```python
from build123d import *

# Parameters (mm, degrees)
SKETCH1_W           = 34
SKETCH1_H           = 30
SKETCH1_R           = 2
BOSS_EXTRUDE1_DEPTH = 22
SKETCH3_R           = 4
CUT_EXTRUDE1_DEPTH  = 30


with BuildPart() as part:
    # Sketch1 → Boss-Extrude1 (new body)
    with BuildSketch(Plane.XY):
        Rectangle(SKETCH1_W, SKETCH1_H)
        with Locations((-12, 9)):
            Circle(SKETCH1_R, mode=Mode.SUBTRACT)
        with Locations((-12, -9)):
            Circle(SKETCH1_R, mode=Mode.SUBTRACT)
        with Locations((12, 9)):
            Circle(SKETCH1_R, mode=Mode.SUBTRACT)
        with Locations((12, -9)):
            Circle(SKETCH1_R, mode=Mode.SUBTRACT)
    extrude(amount=BOSS_EXTRUDE1_DEPTH)

    # Sketch3 → Cut-Extrude1 (cut)
    with BuildSketch(Plane(origin=(0, 15, 0), x_dir=(1, 0, 0), z_dir=(0, 1, 0))):
        with Locations(Location((0, -11, 0), (0, 0, 270))):
            Circle(SKETCH3_R)
        Polygon((-17, -16), (-12, -16), (-6, -22), (-17, -22), align=None)
        Polygon((17, -22), (6, -22), (12, -16), (17, -16), align=None)
        Polygon((-8.5, 0), (-6.414897811, -2.085102189), (6.414897811, -2.085102189), (8.5, 0), align=None)
    extrude(amount=-CUT_EXTRUDE1_DEPTH, mode=Mode.SUBTRACT)


solid = part.part
```
The model under review builds one solid part; all positions refer to its coordinate system, in mm. A direction names the side the tool comes from. Round coordinates to 2 decimals unless told otherwise and drop trailing zeros. Loops run counter-clockwise (first coordinate to the right, second up) from the corner with the lowest first, then second, coordinate; pieces in that order, holes last. Notation, with made-up numbers: (73, -32) -> (91, -32) arc R15 cw to (91, -25) -> close; hole circle Ø10 at (-16, 26.25). An arc over 180 degrees is marked (long way). Answer in a Markdown table with one row per item.
1) Tool access review of faces 1 (the flat face through (-15, 0, 16)), 2 (the flat face through (14, 0, 16)), 3 (the flat face through (0, 0, 22)), 4 (the flat face through (0, 0, 2.085)): name each direction out of +Z, -Z, +X, -X, +Y, -Y from which nothing blocks a thin tool from reaching the whole face with its end or side.
Taken from the geometry:
| item | result |
|---|---|
| face 1 | +Z, -X, +Y, -Y |
| face 2 | +Z, +X, +Y, -Y |
| face 3 | +Z, +X, -X, +Y, -Y |
| face 4 | -Z, +Y, -Y |
2) Consider section D-D, the plane y = 0.5. Write out the cut boundary in (x, z).
Taken from the geometry:
| item | result |
|---|---|
| outline | (-17, 0) -> (-8.5, 0) -> (-6.41, 2.09) -> (6.41, 2.09) -> (8.5, 0) -> (17, 0) -> (17, 16) -> (12, 16) -> (6, 22) -> (-6, 22) -> (-12, 16) -> (-17, 16) -> close; hole circle Ø8 at (0, 11) |
3) Consider section A-A, the plane z = 11. Write out the cut boundary in (x, y).
Taken from the geometry:
| item | result |
|---|---|
| outline | (-17, -15) -> (-4, -15) -> (-4, 15) -> (-17, 15) -> close; (4, -15) -> (17, -15) -> (17, 15) -> (4, 15) -> close; hole circle Ø4 at (-12, -9); hole circle Ø4 at (-12, 9); hole circle Ø4 at (12, -9); hole circle Ø4 at (12, 9) |
4) Consider section C-C, the plane x = -12.5. Write out the cut boundary in (y, z).
Taken from the geometry:
| item | result |
|---|---|
| outline | (-15, 0) -> (-10.94, 0) -> (-10.94, 16) -> (-15, 16) -> close; (-7.06, 0) -> (7.06, 0) -> (7.06, 16) -> (-7.06, 16) -> close; (10.94, 0) -> (15, 0) -> (15, 16) -> (10.94, 16) -> close |
5) Consider section B-B, the plane y = 9. Write out the cut boundary in (x, z), plus the area to 3 significant figures.
Taken from the geometry:
| item | result |
|---|---|
| outline | (-17, 0) -> (-14, 0) -> (-14, 16) -> (-17, 16) -> close; (-10, 0) -> (-8.5, 0) -> (-6.41, 2.09) -> (6.41, 2.09) -> (8.5, 0) -> (10, 0) -> (10, 18) -> (6, 22) -> (-6, 22) -> (-10, 18) -> close; (14, 0) -> (17, 0) -> (17, 16) -> (14, 16) -> close; hole circle Ø8 at (0, 11) |
| area | 439 mm² |
6) For pin 1 Ø4.5 at (x, y) = (-12, -9) entering from -Z; pin 2 Ø3 at (y, z) = (-11.5, 18) entering from +X; pin 3 Ø2 at (y, z) = (4, 19) entering from +X; pin 4 Ø2.5 at (x, y) = (-13.5, -4) entering from +Z, all flat-tipped, find the tip position at first contact; note any pin that passes through.
Taken from the geometry:
| item | result |
|---|---|
| pin 1 | stops at z = 0 |
| pin 2 | stops at x = 11.5 |
| pin 3 | stops at x = 10 |
| pin 4 | stops at z = 16 |
7) Wall thickness on line 1 along X through (y, z) = (-9, 6.25); line 2 along Y through (x, z) = (12, 4.5); line 3 along Y through (x, z) = (-10.5, 12.5): over which ranges is each line inside the solid? List them lowest first.
Taken from the geometry:
| item | result |
|---|---|
| line 1 | x = -17 to -14, -10 to 10, 14 to 17 |
| line 2 | y = -15 to -11, -7 to 7, 11 to 15 |
| line 3 | y = -15 to -10.32, -7.68 to 7.68, 10.32 to 15 |
8) Draft analysis for pull direction X (two halves, no side actions). For faces 5 (the cylindrical face through (10, 9, 9)), 6 (the flat face through (-9, 0, 19)), 7 (the flat face through (17, 0, 8)), state which applies: pulls with the +X half, pulls with the -X half, needs draft (parallel to the pull), parting line crosses it, or undercut.
Taken from the geometry:
| item | result |
|---|---|
| face 5 | undercut |
| face 6 | pulls with the -X half |
| face 7 | pulls with the +X half |
